Build history of the part. All positions in model axes, mm. Round coordinates to 2 decimals unless told otherwise and drop trailing zeros. Write each loop counter-clockwise with the first axis right and the second up, starting at its lowest first coordinate (ties: lowest second). Pieces come first, ordered by that corner, then holes. Notation, with made-up numbers: (33, 59.5) -> (41, 59.5) arc R27 ccw to (41, 92.5) -> close; hole circle Ø3 at (85.25, -28.75). An arc over 180 degrees is marked (long way). Return JSON: item names as keys, results as strings.
from build123d import *

# Parameters (mm, degrees)
F0_R     = 6.5
F0_R_2   = 2
F0_W     = 16
F0_H     = 8
F0_R_3   = 4
F0_R_4   = 1.5
F0_W_2   = 8
F1_DEPTH = 7


with BuildPart() as f1:
    # F0 (on Front) → F1 (new body)
    with BuildSketch(Plane.XZ):
        with BuildLine():
            Line((-113, 0), (0, 0))
            Line((0, 0), (113, 0))
            Line((113, 0), (115, -3))
            Line((115, -3), (195, -3))
            Line((195, -3), (195, 52))
            ThreePointArc((195, 52), (193.535534, 55.535534), (190, 57))
            ThreePointArc((190, 57), (175.857864, 62.857864), (170, 77))
            ThreePointArc((170, 77), (168.535534, 80.535534), (165, 82))
            Line((165, 82), (140, 82))
            ThreePointArc((140, 82), (136.464466, 80.535534), (135, 77))
            Line((135, 77), (135, 46.753148))
            Line((135, 46.753148), (135, 37))
            Line((135, 37), (0, 37))
            Line((0, 37), (-135, 37))
            Line((-135, 37), (-135, 46.753148))
            Line((-135, 46.753148), (-135, 77))
            ThreePointArc((-135, 77), (-136.464466, 80.535534), (-140, 82))
            Line((-140, 82), (-165, 82))
            ThreePointArc((-165, 82), (-168.535534, 80.535534), (-170, 77))
            ThreePointArc((-170, 77), (-175.857864, 62.857864), (-190, 57))
            ThreePointArc((-190, 57), (-193.535534, 55.535534), (-195, 52))
            Line((-195, 52), (-195, -3))
            Line((-195, -3), (-115, -3))
            Line((-115, -3), (-113, 0))
        make_face()
        with Locations((-169.5, 15.5)):
            Circle(F0_R, mode=Mode.SUBTRACT)
        with Locations((-182.5, 34)):
            Circle(F0_R_2, mode=Mode.SUBTRACT)
        with Locations((-169.5, 34)):
            Rectangle(F0_W, F0_H, mode=Mode.SUBTRACT)
        with Locations((-156.5, 34)):
            Circle(F0_R_2, mode=Mode.SUBTRACT)
        with Locations((-97, 19)):
            Circle(F0_R_3, mode=Mode.SUBTRACT)
        with Locations((-44.5, 18.5)):
            Circle(F0_R_4, mode=Mode.SUBTRACT)
        with Locations((169.5, 15.5)):
            Circle(F0_R, mode=Mode.SUBTRACT)
        with Locations((44.5, 18.5)):
            Circle(F0_R_4, mode=Mode.SUBTRACT)
        with Locations((97, 19)):
            Circle(F0_R_3, mode=Mode.SUBTRACT)
        with Locations((156.5, 34)):
            Circle(F0_R_2, mode=Mode.SUBTRACT)
        with Locations((169.5, 34)):
            Rectangle(F0_W, F0_H, mode=Mode.SUBTRACT)
        with Locations((182.5, 34)):
            Circle(F0_R_2, mode=Mode.SUBTRACT)
        with Locations((-150, 46)):
            Rectangle(F0_W_2, F0_H, mode=Mode.SUBTRACT)
        with Locations((-150, 57)):
            Circle(F0_R_2, mode=Mode.SUBTRACT)
        with Locations((-150, 68)):
            Rectangle(F0_W_2, F0_H, mode=Mode.SUBTRACT)
        with Locations((150, 46)):
            Rectangle(F0_W_2, F0_H, mode=Mode.SUBTRACT)
        with Locations((150, 57)):
            Circle(F0_R_2, mode=Mode.SUBTRACT)
        with Locations((150, 68)):
            Rectangle(F0_W_2, F0_H, mode=Mode.SUBTRACT)
    extrude(amount=F1_DEPTH)


solid = f1.part
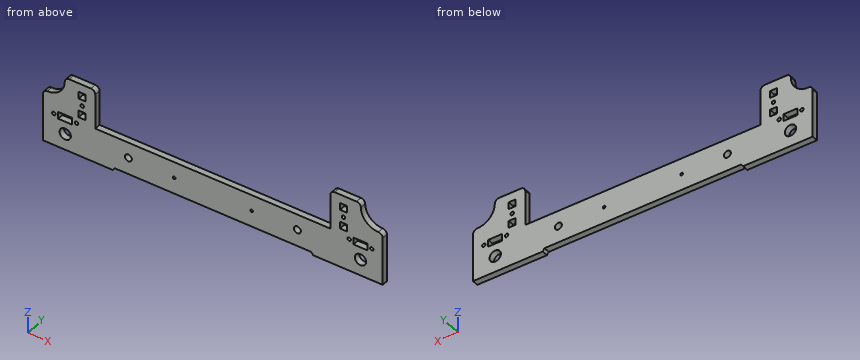
Q1. Saw through at D-D on x = -123.5. List the corners of the cut face in (y, z), then the cut area to 3 significant figures.
Verdict:
{"outline": "(-7, -3) -> (0, -3) -> (0, 37) -> (-7, 37) -> close", "area": "280 mm²"}
Q2. Saw through at B-B on y = -5.25. Count the separate pieces of the cut face and the enclosed holes in it, then the cut area to 3 significant figures.
Verdict:
{"separate pieces": "1", "enclosed holes": "18", "area": "18,200 mm²"}
Q3. Wall check: L1, parallel to Z at x = -150, y = -2.25; L2, parallel to Z at x = -44.5, y = -3; L3, parallel to Z at x = -156.5, y = -1.75. Give the ranges that are in metal, low to high.
Verdict:
{"L1": "z = -3 to 42, 50 to 55, 59 to 64, 72 to 82", "L2": "z = 0 to 17, 20 to 37", "L3": "z = -3 to 32, 36 to 82"}
Q4. Saw through at A-A on x = 97. List the corners of the cut face in (y, z), then the cut area to 3 significant figures.
Verdict:
{"outline": "(-7, 0) -> (0, 0) -> (0, 15) -> (-7, 15) -> close; (-7, 23) -> (0, 23) -> (0, 37) -> (-7, 37) -> close", "area": "203 mm²"}
Q5. Pin check, flat tips, straight feed: pin 1 Ø3.5 at (x, y) = (171, -5) entering from +Z; pin 2 Ø1 at (x, z) = (-113, 12.5) entering from +Y; pin 3 Ø3 at (x, y) = (-103, -5) entering from +Z. Stop position of each tip, or through.
Verdict:
{"pin 1": "stops at z = 79.63", "pin 2": "stops at y = 0", "pin 3": "stops at z = 37"}
Q6. Saw through at C-C on x = -25.5. List the corners of the cut face in (y, z), then the cut area to 3 significant figures.
Verdict:
{"outline": "(-7, 0) -> (0, 0) -> (0, 37) -> (-7, 37) -> close", "area": "259 mm²"}
